```python
from build123d import *

# Parameters (mm, degrees)
F0_W     = 23
F0_H     = 26
F1_DEPTH = 49
F2_R     = 0.1


with BuildPart() as f1:
    # F0 (on Top) → F1 (new body)
    with BuildSketch(Plane.XY):
        Polygon((-24.5, -13), (24.5, -13), (24.5, 13), (-1.5, 13), (-24.5, 13), align=None)
        with Locations((-13, 26)):
            Rectangle(F0_W, F0_H)
    extrude(amount=F1_DEPTH)

    # F2
    f2_edges = [f1.edges().sort_by_distance(p)[0] for p in [
        (0, -13, 49),
        (24.5, 0, 49),
        (11.5, 13, 49),
        (-1.5, 26, 49),
        (-13, 39, 49),
        (-24.5, 13, 49),
        (24.5, -13, 24.5),
        (24.5, 13, 24.5),
        (24.5, 0, 0),
        (11.5, 13, 0),
        (-1.5, 13, 24.5),
        (-1.5, 39, 24.5),
        (-1.5, 26, 0),
        (-24.5, 39, 24.5),
        (-13, 39, 0),
        (-24.5, -13, 24.5),
        (-24.5, 13, 0),
        (0, -13, 0),
    ]]
    fillet(f2_edges, radius=F2_R)


solid = f1.part
```
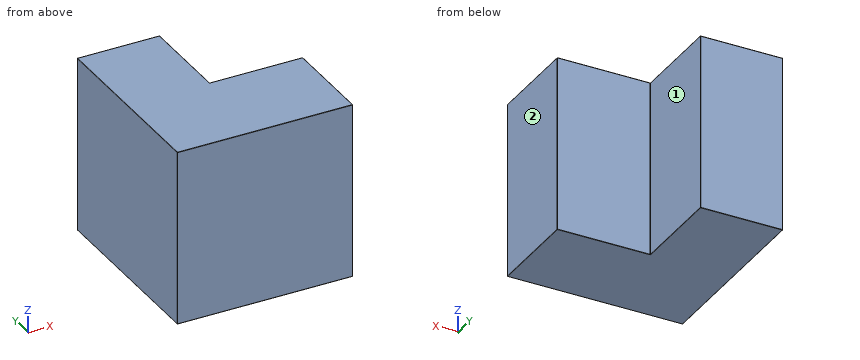
Source: CAD feature listing. Evaluate the final solid. Frame: model axes, mm. Face numbers are marked on the shaded views. A direction names the side the tool comes from. Give positions to 0.01 mm unless a question says otherwise; leave off trailing zeros. Loops run counter-clockwise (first coordinate to the right, second up) from the corner with the lowest first, then second, coordinate; pieces in that order, holes last. Notation, with made-up numbers: (44.25, -3) - (55.25, -3) arc R36 ccw to (55.25, 31) - close; hole circle Ø9 at (80, 10). An arc over 180 degrees is marked (long way). Use CSV: the item, a comma, the result in double quotes.
1) Set-up query: the marked faces 1 and 2. Return all of +Z, -Z, +X, -X, +Y, -Y with unobstructed straight access to the full face (end or side cutting, diameter ignored); none if empty.
Worked out:
face 1,"+Z, -Z, +X, +Y"
face 2,"+Z, -Z, +X, +Y, -Y"
2) Pin query (flat end, axial travel): P1, Ø20.5, axis at y = 24.5, z = 25.5, coming from the +X side; P2, Ø20.5, axis at x = 9, z = 17.5, coming from the +Y side. Return the tip coordinate at first contact, or that it passes through.
Worked out:
P1,"stops at x = -1.5"
P2,"stops at y = 13"
3) Line query: line 1 (Y direction, x = 17, z = 37); line 2 (X direction, y = 19, z = 28.5). Output: solid intervals per line, ascending.
Worked out:
line 1,"y = -13 to 13"
line 2,"x = -24.5 to -1.5"
4) Cut plane B-B (z = 46). Output: boundary loops of the cut face in (x, y).
Worked out:
outline,"(-24.5, -12.9) arc R0.1 ccw to (-24.4, -13) - (24.4, -13) arc R0.1 ccw to (24.5, -12.9) - (24.5, 12.9) arc R0.1 ccw to (24.4, 13) - (-1.4, 13) arc R0.1 cw to (-1.5, 13.1) - (-1.5, 38.9) arc R0.1 ccw to (-1.6, 39) - (-24.4, 39) arc R0.1 ccw to (-24.5, 38.9) - close"
5) Cut plane A-A (y = 24). Output: boundary loops of the cut face in (x, z), and give its area (3 significant figures).
Worked out:
outline,"(-24.5, 0.1) arc R0.1 ccw to (-24.4, 0) - (-1.6, 0) arc R0.1 ccw to (-1.5, 0.1) - (-1.5, 48.9) arc R0.1 ccw to (-1.6, 49) - (-24.4, 49) arc R0.1 ccw to (-24.5, 48.9) - close"
area,"1,130 mm^2"
6) Cut plane C-C (x = 0.5). Output: boundary loops of the cut face in (y, z).
Worked out:
outline,"(-13, 0.1) arc R0.1 ccw to (-12.9, 0) - (12.9, 0) arc R0.1 ccw to (13, 0.1) - (13, 48.9) arc R0.1 ccw to (12.9, 49) - (-12.9, 49) arc R0.1 ccw to (-13, 48.9) - close"
